from build123d import *


with BuildPart() as f1:
    # F0 (on Front) → F1 (revolve)
    with BuildSketch(Plane.XZ):
        with BuildLine():
            Line((75, 0), (75, 6.294016))
            ThreePointArc((75, 6.294016), (343.693177, 159.526249), (450, 450))
            Line((450, 450), (450, 1310))
            ThreePointArc((450, 1310), (343.693177, 1600.473751), (75, 1753.705984))
            Line((75, 1753.705984), (75, 1760))
            Line((75, 1760), (50, 1760))
            Line((50, 1760), (50, 1785))
            Line((50, 1785), (0, 1785))
            Line((0, 1785), (0, 1760))
            Line((0, 1760), (0, 0))
            Line((0, 0), (0, -25))
            Line((0, -25), (50, -25))
            Line((50, -25), (50, 0))
            Line((50, 0), (75, 0))
        make_face()
    revolve(axis=Axis((0, 0, 880), (0, 0, -1)))


solid = f1.part
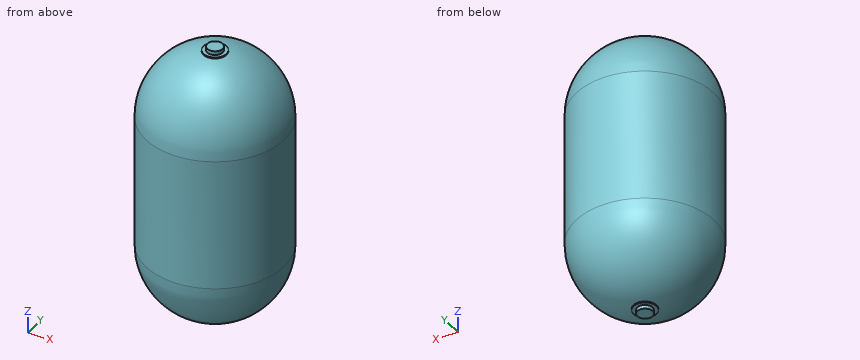
Can you work these out from the model? Positions are in its coordinate system, mm. Coordinates: 2 decimals unless noted, no trailing zeros. Write each loop counter-clockwise with the first axis right and the second up, starting at its lowest first coordinate (ties: lowest second). Pieces come first, ordered by that corner, then holes. Notation, with made-up numbers: M 1.25,62 L 33.25,62 A25 ccw 33.25,87 Z; hole C 35,24.5 d8. An arc over 180 degrees is marked long. Use one line per item in the form item = value.
Q1. For P1, Ø5, axis at x = -25.5, z = 1519, coming from the -Y side; P2, Ø3, axis at x = 225, z = 1030.5, coming from the +Y side; P3, Ø8, axis at x = 347.5, z = 1534.5, coming from the +Y side, each with a flat end and sliding along its axis, tell me the tip position at first contact or that it passes through.
Model answer:
P1 = -399.02
P2 = 390.57
P3 = 186.11
Q2. If we section it at A-A (z = 645): Write out the boundary of the cut face in (x, y), then the cut area to 3 significant figures.
Model answer:
outline = C 0,0 d900
area = 636,000 mm^2
Q3. I need wall thicknesses on line 1 along X through (y, z) = (-168, 1307.5); line 2 along Y through (x, z) = (-359, 436); line 3 along Y through (x, z) = (302, 852.5). Which ranges of each line are inside material? Lowest first, please. Write a range as from..to.
Model answer:
line_1 = -417.46..417.46
line_2 = -270.97..270.97
line_3 = -333.61..333.61
